Autodesk Inventor part; units mm, degrees
ref_plane "YZ Plane" through (0, 0, 0) normal (1, 0, 0) x (0, 1, 0)
ref_plane "XZ Plane" through (0, 0, 0) normal (0, 1, 0) x (-1, 0, 0)
ref_plane "XY Plane" through (0, 0, 0) normal (0, 0, 1) x (1, 0, 0)
sketch "Sketch1" plane through (0, 0, 0) normal (0, 0, 1) x (1, 0, 0)
  line L0 (-184.0318, 0) -> (112.1636, 0)
  line L1 (0, -97.79) -> (0, 97.79)
  circle A0 centre (0, 0) radius 50.8 construction
  arc A1 (-14.6356, -68.2995) -> (-14.6356, 68.2995) centre (0, 0) ccw
  arc A2 (44.9013, -44.9013) -> (57.5505, 26.8363) centre (0, 0) ccw
  arc A3 (40.1305, -40.1305) -> (51.4358, 23.9849) centre (0, 0) ccw
  line L2 (0, 0) -> (57.5505, 26.8363) construction
  line L3 (0, 0) -> (44.9013, -44.9013) construction
  arc A4 (57.5505, 26.8363) -> (51.4358, 23.9849) centre (54.4932, 25.4106) ccw
  arc A5 (40.1305, -40.1305) -> (44.9013, -44.9013) centre (42.5159, -42.5159) ccw
  arc A6 (-101.5622, 49.6724) -> (-101.5622, -49.6724) centre (-90.9182, 0) ccw
  line L4 (-101.5622, 49.6724) -> (-14.6356, 68.2995)
  line L5 (-101.5622, -49.6724) -> (-14.6356, -68.2995)
  circle A7 centre (-74.0404, 25.4) radius 11.1125
  circle A8 centre (-74.0404, -25.4) radius 11.1125
  circle A9 centre (0, 0) radius 19.05
  circle A10 centre (-107.95, 0) radius 14.2875
  line L6 (-107.95, -14.2875) -> (-107.95, 14.2875) construction
  dimension "d0" = 101.6
  dimension "d1" = 19.05
  dimension "d2" = 6.7469
  dimension "d3" = 6.35
  dimension "d4" = 45
  dimension "d5" = 25
  dimension "d10" = 22.225
  dimension "d11" = 38.1
  dimension "d24" = 50.8
  dimension "d33" = 88.9
  dimension "d34" = 107.95
  dimension "d35" = 28.575
extrude "Extrusion1" add sketch "Sketch1" along normal mid plane 6.35 contours A6 L4 A1 L1 A9 L0 A10 | L0 A10 A9 L1 A1 L5 A6 | A1 L0 A2 A4 A3 A9 L1 | L1 A9 L0 A3 A5 A2 A1
sketch "Sketch2" plane through (0, 0, -3.175) normal (0, 0, -1) x (-1, 0, 0)
  line L0 (184.0318, 0) -> (-112.1636, 0)
  line L1 (0, -97.79) -> (0, 97.79)
  point P0 (36.5125, 49.2125)
  point P1 (9.525, -60.325)
  dimension "d15" = 49.2125
  dimension "d16" = 36.5125
  dimension "d39" = 9.525
  dimension "d40" = 60.325
hole "Hole1" at (-36.5125, 49.2125, -3.175) at (-9.525, -60.325, -3.175) direction (0, 0, 1) diameter 5.1054 end through all counterbore diameter 9.779 counterbore depth 1.5875
sketch "Sketch3" plane through (0, 0, -3.175) normal (0, 0, -1) x (-1, 0, 0)
  line L0 (101.5622, -49.6724) -> (101.5622, 49.6724) construction
  line L1 (184.0318, 0) -> (-112.1636, 0)
  line L2 (0, -97.79) -> (0, 97.79)
  point P0 (101.5622, 42.8625)
  point P1 (101.5622, -42.8625)
  dimension "d25" = 42.8625
hole "Hole2" at (-101.5622, 42.8625, -3.175) at (-101.5622, -42.8625, -3.175) direction (0, 0, 1) diameter 5.1054 end through all counterbore diameter 9.779 counterbore depth 1.5875
properties part number "front plate"
Source: CAD feature listing. Evaluate the final solid. Frame: model axes, mm. A direction names the side the tool comes from. Coordinates: 2 decimals unless noted, no trailing zeros. Order: outer loops, then holes, each group sorted by start corner. A loop starts at its lowest first (then second) coordinate and runs counter-clockwise, first axis right, second up. Notation, with made-up numbers: (-26, -8) - (21, -8) arc R12 cw to (21, 6) - close; hole circle Ø5 at (22, -36). An arc over 180 degrees is marked (long way). One line per item, written item: value.
1) Reachability of faces 1 (the face through (62.627, -10.491, -0.044)), 2 (the face through (-37, 1, 3.175)), 3 (the face through (-34, 51, -1.588)) from +Z, -Z, +X, -X, +Y, -Y: full face, straight path, thin tool, end or side. Return the list, or none.
Computed values:
face 1: +Z, -Z
face 2: +Z, +X, -X, +Y, -Y
face 3: -Z
2) Ray query, line 1 (X direction, y = 0, z = 1.5); line 2 (X direction, y = 10, z = 0.5); line 3 (Y direction, x = -70.5, z = 2). Return the intervals inside material, ascending. Write a range as [from, to].
Computed values:
line 1: x = [-141.72, -122.24], [-93.66, -19.05], [19.05, 56.75], [63.5, 69.85]
line 2: x = [-140.72, -118.15], [-97.75, -16.21], [16.21, 55.87], [62.71, 69.13]
line 3: y = [-56.33, -35.93], [-14.87, 14.87], [35.93, 56.33]
3) Cut plane B-B on x = 0. Output: boundary loops of the cut face in (y, z) (3 decimals), plus the area to 3 significant figures.
Computed values:
outline: (-69.85, -3.175) - (-19.05, -3.175) - (-19.05, 3.175) - (-69.85, 3.175) - close; (19.05, -3.175) - (69.85, -3.175) - (69.85, 3.175) - (19.05, 3.175) - close
area: 645 mm^2
4) Cut plane A-A on y = 0. State how many separate pieces and enclosed holes the cut face has, plus the area to 3 significant figures.
Computed values:
separate pieces: 4
enclosed holes: 0
area: 877 mm^2
5) Cut plane D-D on y = -25.4. Output: boundary loops of the cut face in (x, z) (3 decimals).
Computed values:
outline: (-134.912, -3.175) - (-85.153, -3.175) - (-85.153, 3.175) - (-134.912, 3.175) - close; (-62.928, -3.175) - (50.752, -3.175) - (50.752, 3.175) - (-62.928, 3.175) - close; (58.199, -3.175) - (65.068, -3.175) - (65.068, 3.175) - (58.199, 3.175) - close
6) Mould query, pull axis Y, two halves, no side actions, for faces 4 (the face through (-141.71, -0.97, -0.04)), 5 (the face through (-7.97, -62.35, 0.83)), 6 (the face through (-58.707, -58.856, -0.044)). Classes: released by +Y, released by -Y, zero draft, split by the parting line, or undercut.
Computed values:
face 4: split by the parting line
face 5: undercut
face 6: released by -Y
7) Contact query for flat-ended pins moving along their axis: pin 1 (9 mm diameter, centred on x = -101.56, y = -42.86, fed in from -Z); pin 2 (20 mm diameter, centred on x = -74.04, y = 25.4, fed in from +Z). Output: stop coordinate, or through.
Computed values:
pin 1: stops at z = -1.59
pin 2: passes through
